Print and shaded views of the part. All mm, measured from the part's lowest x, y and z. Coordinates: 2 decimals unless noted, no trailing zeros. Loops run counter-clockwise (first coordinate to the right, second up) from the corner with the lowest first, then second, coordinate; pieces in that order, holes last. Notation, with made-up numbers: M 24,74 L 58,74 A16 ccw 58,91 Z; hole C 44,26.5 d7. An arc over 180 degrees is marked long. One line per question, with ' | ' between items. Start each with the question number.
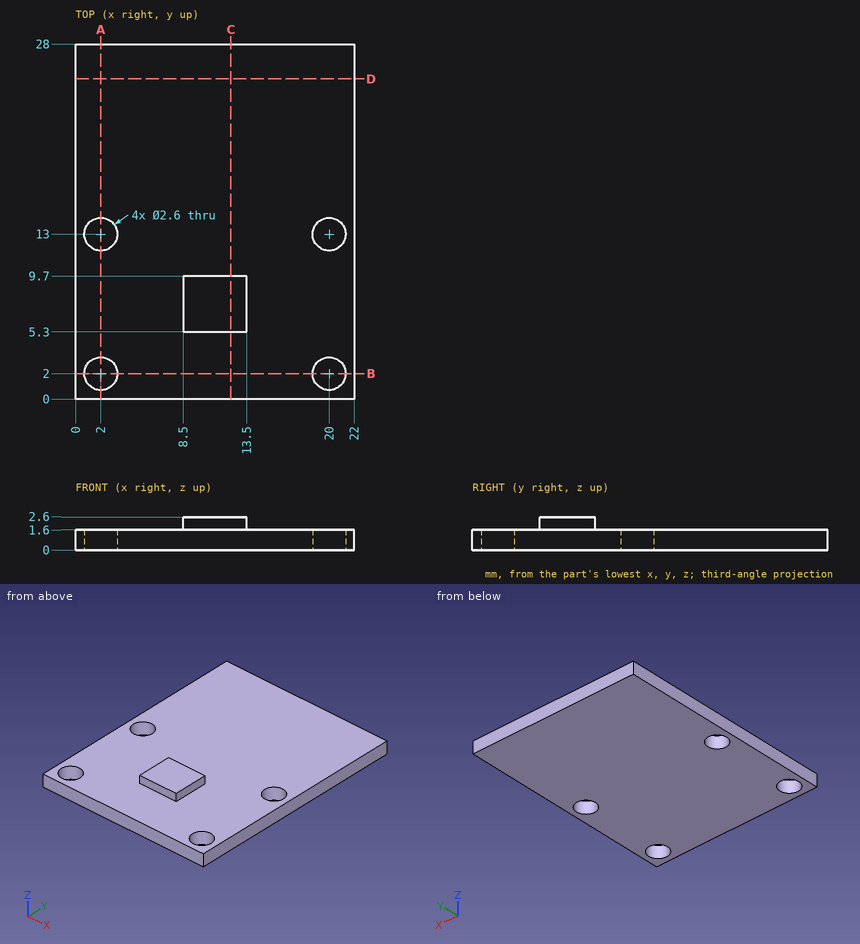
(1) Band-saw the part on C-C on x = 12.25. Write the cut outline in (y, z).
(2) Band-saw the part on A-A on x = 2. Write the cut outline in (y, z).
(3) Band-saw the part on B-B on y = 2. Write the cut outline in (x, z), then the cut area to 3 significant figures.
(4) Band-saw the part on D-D on y = 25.25. Write the cut outline in (x, z), then the cut area to 3 significant figures.
(5) Drill centre lines: line 1 (X direction, y = 13, z = 0.6); line 2 (Y direction, x = 20, z = 0.95); line 3 (Z direction, x = 11.75, y = 23.25). Where is each one in solid material? Low to high. Write a range as [from, to].
(6) Pin check, flat tips, straight feed: P1, Ø4, axis at x = 4.5, y = 18.5, coming from the +Z side; P2, Ø3, axis at x = 20, y = 13, coming from the -Z side; P3, Ø1.1, axis at y = 8, z = 2.5, coming from the -X side; P4, Ø1.6, axis at x = 2, y = 2, coming from the -Z side. Stop position of each tip, or through.
Computed values:
1) outline: M 0,0 L 28,0 L 28,1.6 L 9.7,1.6 L 9.7,2.6 L 5.3,2.6 L 5.3,1.6 L 0,1.6 Z
2) outline: M 0,0 L 0.7,0 L 0.7,1.6 L 0,1.6 Z; M 3.3,0 L 11.7,0 L 11.7,1.6 L 3.3,1.6 Z; M 14.3,0 L 28,0 L 28,1.6 L 14.3,1.6 Z
3) outline: M 0,0 L 0.7,0 L 0.7,1.6 L 0,1.6 Z; M 3.3,0 L 18.7,0 L 18.7,1.6 L 3.3,1.6 Z; M 21.3,0 L 22,0 L 22,1.6 L 21.3,1.6 Z | area: 26.9 mm^2
4) outline: M 0,0 L 22,0 L 22,1.6 L 0,1.6 Z | area: 35.2 mm^2
5) line 1: [0, 0.7], [3.3, 18.7], [21.3, 22] | line 2: [0, 0.7], [3.3, 11.7], [14.3, 28] | line 3: [0, 1.6]
6) P1: z = 1.6 | P2: z = 0 | P3: x = 8.5 | P4: through
